from build123d import *

# Parameters (mm, degrees)
SKETCH1_R           = 4
BOSS_EXTRUDE1_DEPTH = 5


with BuildPart() as part:
    # Sketch1 → Boss-Extrude1 (new body)
    with BuildSketch(Plane.XY):
        with BuildLine():
            Line((-29.957010387, -40.140273422), (-29.957010387, -45.140273422))
            Line((-29.957010387, -45.140273422), (-14.957010387, -45.140273422))
            Line((-14.957010387, -45.140273422), (-14.957010387, -40.140273422))
            Line((-14.957010387, -40.140273422), (-1.457010387, -40.140273422))
            Line((-1.457010387, -40.140273422), (-1.457010387, -29.140273422))
            Line((-1.457010387, -29.140273422), (-2.757010387, -29.140273422))
            Line((-2.757010387, -29.140273422), (-2.757010387, -26.640273422))
            Line((-2.757010387, -26.640273422), (-1.457010387, -26.640273422))
            Line((-1.457010387, -26.640273422), (-1.457010387, -19.640273422))
            Line((-1.457010387, -19.640273422), (1.542989613, -19.640273422))
            Line((1.542989613, -19.640273422), (1.542989613, -26.640273422))
            Line((1.542989613, -26.640273422), (2.842989613, -26.640273422))
            Line((2.842989613, -26.640273422), (2.842989613, -29.140273422))
            Line((2.842989613, -29.140273422), (1.542989613, -29.140273422))
            Line((1.542989613, -29.140273422), (1.542989613, -40.140273422))
            Line((1.542989613, -40.140273422), (15.042989613, -40.140273422))
            Line((15.042989613, -40.140273422), (15.042989613, -45.140273422))
            Line((15.042989613, -45.140273422), (30.042989613, -45.140273422))
            Line((30.042989613, -45.140273422), (30.042989613, -40.140273422))
            Line((30.042989613, -40.140273422), (90.042989613, -40.140273422))
            Line((90.042989613, -40.140273422), (62.323763373, 89.216115695))
            ThreePointArc((62.323763373, 89.216115695), (57.728251424, 95.673109145), (49.877526115, 96.75828499))
            add(Edge.make_bspline(
                [(49.877526115, 96.75828499), (33.266013947, 92.159246048), (0.042989613, 87.560207107), (-33.180034722, 92.159246048), (-49.791546889, 96.75828499)],
                knots=[0.084712196, 0.084712196, 0.084712196, 0.084712196, 0.5, 0.915287804, 0.915287804, 0.915287804, 0.915287804], degree=3))
            ThreePointArc((-49.791546889, 96.75828499), (-57.642272198, 95.673109145), (-62.237784148, 89.216115695))
            Line((-62.237784148, 89.216115695), (-89.957010387, -40.140273422))
            Line((-89.957010387, -40.140273422), (-29.957010387, -40.140273422))
        make_face()
        with Locations((26.442989613, 59.859726578)):
            Circle(SKETCH1_R, mode=Mode.SUBTRACT)
        with Locations((0.042989613, 59.859726578)):
            Circle(SKETCH1_R, mode=Mode.SUBTRACT)
    extrude(amount=BOSS_EXTRUDE1_DEPTH)


solid = part.part
Geometry check sheet. Reference: the model listing, model coordinates, mm. A direction names the side the tool comes from. Coordinates: 2 decimals unless noted, no trailing zeros. Order: outer loops, then holes, each group sorted by start corner. A loop starts at its lowest first (then second) coordinate and runs counter-clockwise, first axis right, second up. Notation, with made-up numbers: (6, 62) -> (58, 62) arc R31 ccw to (58, 94) -> close; hole circle Ø2 at (9, -5.75). An arc over 180 degrees is marked (long way). Use a Markdown table: item, result. Add a question column.
1. Cross-section at D-D (z = 2.05). Give the number of separate pieces and of enclosed holes in the cut face, and give its area (3 significant figures).
2. Cross-section at C-C (x = 67.5). Enter the section's corners in (y, z), and give its area (3 significant figures).
3. Set-up check for faces 1 (the face through (-60, -40.14, 2)), 2 (the face through (1.543, -23, 2)), 3 (the face through (30.043, -43, 2)): record each of +Z, -Z, +X, -X, +Y, -Y from which the full face is reachable in a straight line by a thin tool's end or side.
4. Cross-section at B-B (y = -32.5). Enter the section's corners in (x, z).
5. Mould release check, pull along X, two halves, no side actions. Record for faces 4 (the face through (-8, -40.14, 2)), 5 (the face through (-23, -45.14, 2)), 6 (the face through (-29.957, -43, 2)): pulls with the +X half, pulls with the -X half, needs draft (parallel to the pull), parting line crosses it, or undercut.
6. Cross-section at A-A (y = 58). Enter the section's corners in (x, z).
7. Material ranges on L1, parallel to X at y = 61.5, z = 2.75; L2, parallel to Y at x = -52, z = 0.65; L3, parallel to Y at x = 27.5, z = 3.1, recorded low to high.
8. Go/stop test with flat-tipped pins: pin 1 Ø0.9 at (x, z) = (0.5, 3) entering from -Y; pin 2 Ø2.5 at (y, z) = (-24, 3) entering from +X; pin 3 Ø1.5 at (y, z) = (50.5, 0.5) entering from +X. Record where each tip stops, or that it passes through.
Filled sheet:
| question | item | result |
|---|---|---|
| 1 | separate pieces | 1 |
| 1 | enclosed holes | 2 |
| 1 | area | 20,100 mm2 |
| 2 | outline | (-40.14, 0) -> (65.06, 0) -> (65.06, 5) -> (-40.14, 5) -> close |
| 2 | area | 526 mm2 |
| 3 | face 1 | +Z, -Z, -X, -Y |
| 3 | face 2 | +Z, -Z, -Y |
| 3 | face 3 | +Z, -Z, +X, -Y |
| 4 | outline | (-88.32, 0) -> (-1.46, 0) -> (-1.46, 5) -> (-88.32, 5) -> close; (1.54, 0) -> (88.41, 0) -> (88.41, 5) -> (1.54, 5) -> close |
| 5 | face 4 | undercut |
| 5 | face 5 | needs draft |
| 5 | face 6 | pulls with the -X half |
| 6 | outline | (-68.93, 0) -> (-3.5, 0) -> (-3.5, 5) -> (-68.93, 5) -> close; (3.58, 0) -> (22.9, 0) -> (22.9, 5) -> (3.58, 5) -> close; (29.98, 0) -> (69.01, 0) -> (69.01, 5) -> (29.98, 5) -> close |
| 7 | L1 | -68.18 to -3.61, 3.69 to 22.79, 30.09 to 68.26 |
| 7 | L2 | -40.14 to 97.11 |
| 7 | L3 | -45.14 to 56, 63.72 to 91.95 |
| 8 | pin 1 | y = -19.64 |
| 8 | pin 2 | x = 86.85 |
| 8 | pin 3 | x = 70.78 |
